The figure shows three views and two pictorial views of one solid part (mm, origin at its lowest corner). Answer the questions. A direction names the side the tool comes from. Coordinates: 2 decimals unless noted, no trailing zeros. Loops run counter-clockwise (first coordinate to the right, second up) from the corner with the lowest first, then second, coordinate; pieces in that order, holes last. Notation, with made-up numbers: (79.25, 59) -> (115.25, 59) arc R19 cw to (115.25, 64) -> close; hole circle Ø2 at (65.5, 63). An arc over 180 degrees is marked (long way). Use a Markdown table: item, result. Add a question column.
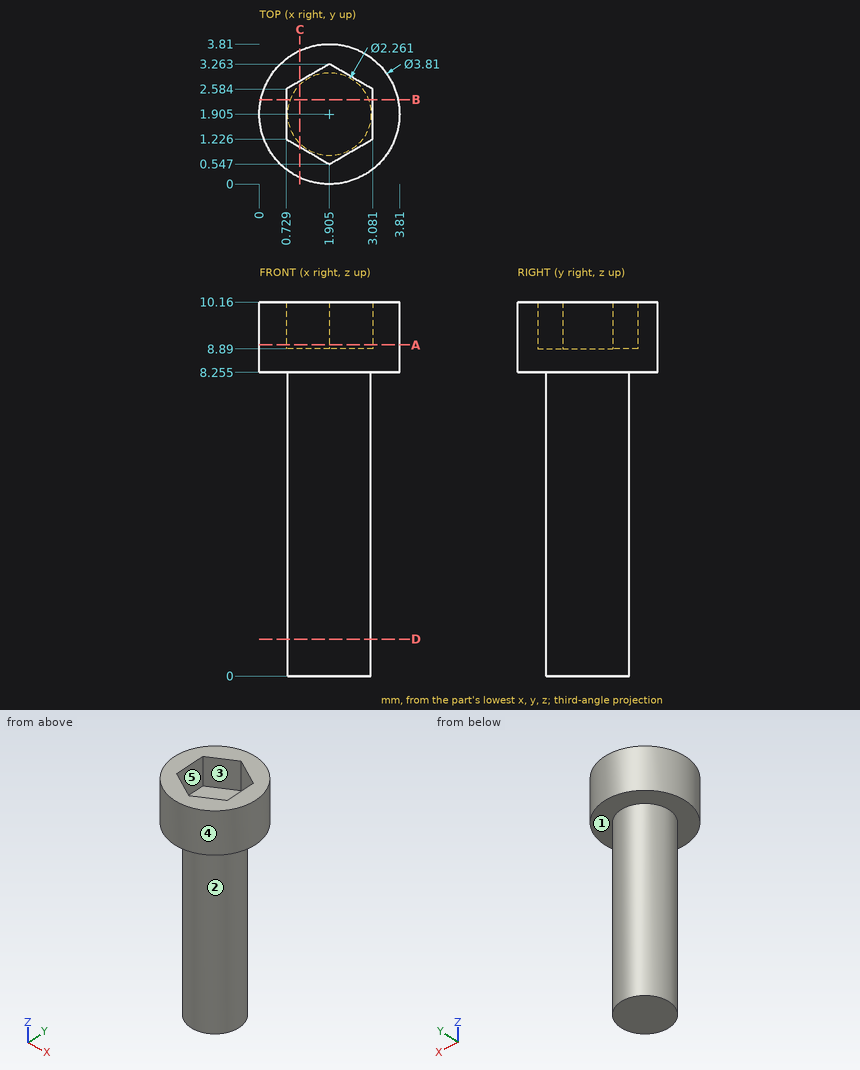
Item 1: Section B-B (y = 2.3) is taken. Determine the outline of the cut face in (x, z) (1 decimal), then the cut area to 3 significant figures.
Item 2: Section C-C (x = 1.1) is taken. Determine the outline of the cut face in (y, z) (1 decimal).
Item 3: Find the intervals of material crossed by probe 1 along Z at (x, y) = (1.2, 1.6); probe 2 along Y at (x, z) = (1.9, 1) (1 decimal); probe 3 along Z at (x, y) = (1.5, 0.4) (1 decimal), in increasing order.
Item 4: Given pin 1 (2 mm diameter, centred on x = 1, y = 2, fed in from -Z); pin 2 (2 mm diameter, centred on y = 1, z = 1.5, fed in from -X) (1 decimal); pin 3 (0.6 mm diameter, centred on y = 1.5, z = 10, fed in from -X); pin 4 (2 mm diameter, centred on y = 1.5, z = 7, fed in from +X) (1 decimal), each flat-ended and moving along its own axis, determine where each tip first touches the part or whether it passes through.
Item 5: For the marked faces 4 and 5, determine the directions among +Z, -Z, +X, -X, +Y, -Y from which every point of the face is accessible in a straight line to the end or side of a thin tool.
Item 6: Section D-D (z = 1) is taken. Determine the outline of the cut face in (x, y) (1 decimal).
Item 7: For a pull along X with two mould halves and no side action, classify the marked faces 1, 2 and 3 as +X half, -X half, draft (parallel to the pull), parting line (faces both ways), or undercut.
Item 8: Section A-A (z = 9) is taken. Determine the outline of the cut face in (x, y) (1 decimal).
Output:
| question | item | result |
|---|---|---|
| 1 | outline | (0, 8.3) -> (0.8, 8.3) -> (0.8, 0) -> (3, 0) -> (3, 8.3) -> (3.8, 8.3) -> (3.8, 10.2) -> (3.1, 10.2) -> (3.1, 8.9) -> (0.7, 8.9) -> (0.7, 10.2) -> (0, 10.2) -> close |
| 1 | area | 21.6 mm2 |
| 2 | outline | (0.2, 8.3) -> (1.1, 8.3) -> (1.1, 0) -> (2.7, 0) -> (2.7, 8.3) -> (3.6, 8.3) -> (3.6, 10.2) -> (2.8, 10.2) -> (2.8, 8.9) -> (1, 8.9) -> (1, 10.2) -> (0.2, 10.2) -> close |
| 3 | probe 1 | z = 0 to 8.89 |
| 3 | probe 2 | y = 0.8 to 3 |
| 3 | probe 3 | z = 8.3 to 10.2 |
| 4 | pin 1 | stops at z = 0 |
| 4 | pin 2 | stops at x = 0.8 |
| 4 | pin 3 | stops at x = 0 |
| 4 | pin 4 | stops at x = 3 |
| 5 | face 4 | +Z, -Z |
| 5 | face 5 | +Z |
| 6 | outline | circle Ø2.3 at (1.9, 1.9) |
| 7 | face 1 | draft |
| 7 | face 2 | parting line |
| 7 | face 3 | undercut |
| 8 | outline | circle Ø3.8 at (1.9, 1.9); hole (0.7, 1.2) -> (1.9, 0.5) -> (3.1, 1.2) -> (3.1, 2.6) -> (1.9, 3.3) -> (0.7, 2.6) -> close |
